Design review of the part built by this model. Coordinates are the model's own, in mm. A direction names the side the tool comes from. Coordinates: 2 decimals unless noted, no trailing zeros. Order: outer loops, then holes, each group sorted by start corner. A loop starts at its lowest first (then second) coordinate and runs counter-clockwise, first axis right, second up. Notation, with made-up numbers: M 62.5,52.5 L 100.5,52.5 A27 ccw 100.5,84.5 Z; hole C 13,29 d5. An arc over 180 degrees is marked long. Answer as a JSON object with one key per item and string values.
from build123d import *

# Parameters (mm, degrees)
EXTRUDE_1_DEPTH     = 15
SKETCH_2_R          = 5.5
EXTRUDE_2_DEPTH     = 5.7
SKETCH_3_R          = 4.25
CUT_EXTRUDE_1_DEPTH = 12.7
M8X1_25_1_D         = 8
SKETCH_8_W          = 0.5
SKETCH_8_H          = 1


with BuildPart() as part:
    # 草图1 → 凸台-拉伸1 (new body)
    with BuildSketch(Plane.XY):
        Polygon((-8.082903769, 0), (-4.041451884, -7), (4.041451884, -7), (8.082903769, 0), (4.041451884, 7), (-4.041451884, 7), align=None)
    extrude(amount=EXTRUDE_1_DEPTH)

    # 草图2 → 凸台-拉伸2 (add)
    with BuildSketch(Plane.XY.offset(15)):
        Circle(SKETCH_2_R)
    extrude(amount=EXTRUDE_2_DEPTH)

    # 草图3 → 切除-拉伸1 (cut)
    with BuildSketch(Plane.XY.offset(20.7)):
        Circle(SKETCH_3_R)
    extrude(amount=-CUT_EXTRUDE_1_DEPTH, mode=Mode.SUBTRACT)

    # M8x1.25 螺纹孔1 (through all)
    with Locations(Plane(origin=(0, 0, 0), x_dir=(-1, 0, 0), z_dir=(0, 0, -1))):
        with Locations((0, 0)):
            Hole(M8X1_25_1_D / 2)

    # 草图8 → 切除-旋转1 (revolve, cut)
    with BuildSketch(Plane(origin=(0, 0, 0), x_dir=(1, 0, 0), z_dir=(0, 1, 0)), mode=Mode.PRIVATE) as cut_revolve_1_sk:
        with Locations((-5.25, -17.7)):
            Rectangle(SKETCH_8_W, SKETCH_8_H)
    revolve(cut_revolve_1_sk.sketch.rotate(Axis((0, 0, 8), (0, 0, -1)), 180), axis=Axis((0, 0, 8), (0, 0, -1)), mode=Mode.SUBTRACT)

    # 草图9 → 切除-旋转2 (revolve, cut)
    with BuildSketch(Plane(origin=(0, 0, 0), x_dir=(1, 0, 0), z_dir=(0, 1, 0))):
        with BuildLine():
            Line((-8.082903769, -1.5), (-8.082903769, 0))
            Line((-8.082903769, 0), (-6.582903769, 0))
            ThreePointArc((-6.582903769, 0), (-7.64356394, -0.439339828), (-8.082903769, -1.5))
        make_face()
    revolve(axis=Axis((0, 0, 8), (0, 0, -1)), mode=Mode.SUBTRACT)


solid = part.part
1) Insertion check: pin 1 Ø2 at (y, z) = (2, 2.5) entering from +X; pin 2 Ø5.5 at (x, y) = (0.5, -0.5) entering from +Z; pin 3 Ø8 at (y, z) = (5, 15.5) entering from -X; pin 4 Ø6 at (y, z) = (-5.5, 11) entering from +X. Each pin has a flat end and moves straight along its axis. Give the tip position at first contact, or say it passes through.
Taken from the geometry:
{"pin 1": "stops at x = 7.51", "pin 2": "passes through", "pin 3": "stops at x = -7.49", "pin 4": "stops at x = 6.64"}
2) Tool access review of faces 5 (the cylindrical face through (2.285, 3.584, 14.439)), 6 (the flat face through (1.6, 4.9, 18.2)), 7 (the flat face through (0, 7, 7)): name each direction out of +Z, -Z, +X, -X, +Y, -Y from which nothing blocks a thin tool from reaching the whole face with its end or side.
Taken from the geometry:
{"face 5": "+Z", "face 6": "none", "face 7": "+Z, -Z, +X, -X, +Y"}
3) Add section C-C (z = 16.5). State the section outline as (x, y) points.
Taken from the geometry:
{"outline": "C 0,0 d11; hole C 0,0 d8.5"}
4) Mouldability with a two-part tool opening along Z and no side actions: class faces 1 (the flat face through (1.6, 4.9, 17.2)), 2 (the flat face through (3, -3, 0)), 3 (the flat face through (0, -7, 7)), 4 (the flat face through (3, 5, 15)) as released by +Z, released by -Z, zero draft, split by the parting line, or undercut.
Taken from the geometry:
{"face 1": "undercut", "face 2": "released by -Z", "face 3": "zero draft", "face 4": "released by +Z"}
5) Add section A-A (z = 14.25). State the section outline as (x, y) points, and give its area (3 significant figures).
Taken from the geometry:
{"outline": "M -8.08,0 L -4.04,-7 L 4.04,-7 L 8.08,0 L 4.04,7 L -4.04,7 Z; hole C 0,0 d8.5", "area": "113 mm2"}
6) Add section B-B (x = 0). State the section outline as (y, z) points.
Taken from the geometry:
{"outline": "M -7,0.06 A1.5 ccw -6.58,0 L -4,0 L -4,8 L -4.25,8 L -4.25,20.7 L -5.5,20.7 L -5.5,18.2 L -5,18.2 L -5,17.2 L -5.5,17.2 L -5.5,15 L -7,15 Z; M 4,0 L 6.58,0 A1.5 ccw 7,0.06 L 7,15 L 5.5,15 L 5.5,17.2 L 5,17.2 L 5,18.2 L 5.5,18.2 L 5.5,20.7 L 4.25,20.7 L 4.25,8 L 4,8 Z"}
7) To check wall thickness, follow L1, parallel to Y at x = 0, z = 5; L2, parallel to Y at x = 0, z = 11; L3, parallel to Z at x = 4.25, y = -3.25. State the ranges of each line that lie inside material, in increasing order.
Taken from the geometry:
{"L1": "y = -7 to -4, 4 to 7", "L2": "y = -7 to -4.25, 4.25 to 7", "L3": "z = 0 to 17.2, 18.2 to 20.7"}
